from build123d import *

# Parameters (mm, degrees)
SKETCH1_W           = 42
SKETCH1_H           = 62
SKETCH1_R           = 11.5
BOSS_EXTRUDE1_DEPTH = 10
FILLET2_R           = 3
SKETCH2_R           = 1.5
CUT_EXTRUDE1_DEPTH  = 11
SKETCH3_R           = 2.6
CUT_EXTRUDE2_DEPTH  = 11


with BuildPart() as part:
    # Sketch1 → Boss-Extrude1 (new body)
    with BuildSketch(Plane.XY):
        with Locations((21, 31)):
            Rectangle(SKETCH1_W, SKETCH1_H)
        with Locations((21, 42)):
            Circle(SKETCH1_R, mode=Mode.SUBTRACT)
    extrude(amount=BOSS_EXTRUDE1_DEPTH)

    # Fillet2
    fillet2_edges = [part.edges().sort_by_distance(p)[0] for p in [
        (0, 62, 5),
        (42, 62, 5),
    ]]
    fillet(fillet2_edges, radius=FILLET2_R)

    # Sketch2 → Cut-Extrude1 (cut, through all)
    with BuildSketch(Plane.XY.offset(10)):
        with Locations((5.5, 57.5)):
            Circle(SKETCH2_R)
        with Locations((36.5, 57.5)):
            Circle(SKETCH2_R)
        with Locations((5.5, 26.5)):
            Circle(SKETCH2_R)
        with Locations((36.5, 26.5)):
            Circle(SKETCH2_R)
    extrude(amount=-CUT_EXTRUDE1_DEPTH, mode=Mode.SUBTRACT)

    # Sketch3 → Cut-Extrude2 (cut, through all)
    with BuildSketch(Plane.XY.offset(10)):
        with Locations((5, 7.5)):
            Circle(SKETCH3_R)
        with Locations((21, 7.5)):
            Circle(SKETCH3_R)
        with Locations((37, 7.5)):
            Circle(SKETCH3_R)
    extrude(amount=-CUT_EXTRUDE2_DEPTH, mode=Mode.SUBTRACT)


solid = part.part
Design review of the part built by this model. Coordinates are the model's own, in mm. Coordinates: 2 decimals unless noted, no trailing zeros. Order: outer loops, then holes, each group sorted by start corner. A loop starts at its lowest first (then second) coordinate and runs counter-clockwise, first axis right, second up. Notation, with made-up numbers: (44.5, -25.5) -> (84.5, -25.5) arc R13 cw to (84.5, -18.5) -> close; hole circle Ø8 at (58.5, -6.75). An arc over 180 degrees is marked (long way). Use one line per item in the form item = value. Start each with the question number.
(1) Add section C-C on y = 57.5. State the section outline as (x, z) points.
(2) Add section A-A on y = 42. State the section outline as (x, z) points, plus the area to 3 significant figures.
(3) Add section B-B on x = 21. State the section outline as (y, z) points.
(4) The part is to be moulded in two halves that separate along Y. For faces 1 (the flat face through (0, 29, 5)), 2 (the flat face through (21, 62, 5)), 3 (the flat face through (21, 0, 5)), 4 (the cylindrical face through (35.39, 58.51, 5.07)), say which applies: +Y half, -Y half, draft (parallel to the pull), parting line (faces both ways), or undercut.
(5) Add section D-D on z = 1.25. Give the number of separate pieces and of enclosed holes in the cut face, plus the area to 3 significant figures.
(6) For probe 1 along Y at (x, z) = (36.5, 2.25); probe 2 along X at (y, z) = (47, 6.25); probe 3 along X at (y, z) = (37.5, 7.5), list the stretches that pass through material, from the lowest coordinate up.
(7) Insertion check: pin 1 (8 mm diameter, centred on x = 12.5, y = 21.5, fed in from -Z). The pin has a flat end and moves straight along its axis. Give the tip position at first contact, or say it passes through.
Answer block:
q1.outline = (0, 0) -> (4, 0) -> (4, 10) -> (0, 10) -> close; (7, 0) -> (35, 0) -> (35, 10) -> (7, 10) -> close; (38, 0) -> (42, 0) -> (42, 10) -> (38, 10) -> close
q2.outline = (0, 0) -> (9.5, 0) -> (9.5, 10) -> (0, 10) -> close; (32.5, 0) -> (42, 0) -> (42, 10) -> (32.5, 10) -> close
q2.area = 190 mm²
q3.outline = (0, 0) -> (4.9, 0) -> (4.9, 10) -> (0, 10) -> close; (10.1, 0) -> (30.5, 0) -> (30.5, 10) -> (10.1, 10) -> close; (53.5, 0) -> (62, 0) -> (62, 10) -> (53.5, 10) -> close
q4.face_1 = draft
q4.face_2 = +Y half
q4.face_3 = -Y half
q4.face_4 = undercut
q5.separate_pieces = 1
q5.enclosed_holes = 8
q5.area = 2,090 mm²
q6.probe_1 = 0 to 4.95, 10.05 to 25, 28 to 56, 59 to 62
q6.probe_2 = 0 to 10.64, 31.36 to 42
q6.probe_3 = 0 to 10.42, 31.58 to 42
q7.pin_1 = 0
